```python
from build123d import *

# Parameters (mm, degrees)
SKETCH1_R               = 33
SKETCH1_R_2             = 25.5
BOSS_EXTRUDE2_DEPTH     = 17
BOSS_EXTRUDE3_START     = -5
SKETCH1_3_R             = 33
BOSS_EXTRUDE3_DEPTH     = 5
CUT_EXTRUDE4_DEPTH      = 50.668903753
CUT_EXTRUDE4_DEPTH_BACK = 3
SKETCH1_5_R             = 1.5
CUT_EXTRUDE6_DEPTH      = 50.668903753
CUT_EXTRUDE6_DEPTH_BACK = 50.668903753
SKETCH3_R               = 1.7
SKETCH3_R_2             = 3.5
SKETCH4_R               = 10
CUT_EXTRUDE7_DEPTH      = 2
SKETCH6_R               = 1.7
CUT_EXTRUDE8_DEPTH      = 10
SKETCH7_R               = 2.75
CUT_EXTRUDE9_DEPTH      = 2


with BuildPart() as part:
    # Sketch1 → Boss-Extrude2 (new body)
    with BuildSketch(Plane.XY):
        Circle(SKETCH1_R)
        Circle(SKETCH1_R_2, mode=Mode.SUBTRACT)
    extrude(amount=BOSS_EXTRUDE2_DEPTH)

    # Sketch1<3> → Boss-Extrude3 (add)
    with BuildSketch(Plane.XY.offset(BOSS_EXTRUDE3_START)):
        Circle(SKETCH1_3_R)
    extrude(amount=BOSS_EXTRUDE3_DEPTH)

    # Sketch1<5> → Cut-Extrude4 (cut, two sides: drawn at the far end of the back side and taken through both)
    with BuildSketch(Plane.XY.offset(-CUT_EXTRUDE4_DEPTH_BACK)):
        with Locations(Location((25, 0, 0), (0, 0, 72.141537302))):
            Circle(SKETCH1_5_R)
        with Locations(Location((24.273545436, -5.982891607, 0), (0, 0, 274.012308852))):
            Circle(SKETCH1_5_R)
        with Locations(Location((22.136400641, -11.618079301, 0), (0, 0, 260.166155006))):
            Circle(SKETCH1_5_R)
        with Locations(Location((18.712768704, -16.578066456, 0), (0, 0, 246.32000116))):
            Circle(SKETCH1_5_R)
        with Locations(Location((14.201618668, -20.574596647, 0), (0, 0, 232.473847314))):
            Circle(SKETCH1_5_R)
        with Locations(Location((8.865122176, -23.375406067, 0), (0, 0, 218.627693468))):
            Circle(SKETCH1_5_R)
        with Locations(Location((3.013417006, -24.817721852, 0), (0, 0, 204.781539621))):
            Circle(SKETCH1_5_R)
        with Locations(Location((-3.013417006, -24.817721852, 0), (0, 0, 190.935385775))):
            Circle(SKETCH1_5_R)
        with Locations(Location((-8.865122176, -23.375406067, 0), (0, 0, 177.089231929))):
            Circle(SKETCH1_5_R)
        with Locations(Location((-14.201618668, -20.574596647, 0), (0, 0, 163.243078083))):
            Circle(SKETCH1_5_R)
        with Locations(Location((-18.712768704, -16.578066456, 0), (0, 0, 149.396924237))):
            Circle(SKETCH1_5_R)
        with Locations(Location((-22.136400641, -11.618079301, 0), (0, 0, 135.550770391))):
            Circle(SKETCH1_5_R)
        with Locations(Location((-24.273545436, -5.982891607, 0), (0, 0, 121.704616545))):
            Circle(SKETCH1_5_R)
        with Locations(Location((-25, 0, 0), (0, 0, 107.858462698))):
            Circle(SKETCH1_5_R)
        with Locations(Location((-24.273545436, 5.982891607, 0), (0, 0, 238.295383455))):
            Circle(SKETCH1_5_R)
        with Locations(Location((-22.136400641, 11.618079301, 0), (0, 0, 224.449229609))):
            Circle(SKETCH1_5_R)
        with Locations(Location((-18.712768704, 16.578066456, 0), (0, 0, 210.603075763))):
            Circle(SKETCH1_5_R)
        with Locations(Location((-14.201618668, 20.574596647, 0), (0, 0, 196.756921917))):
            Circle(SKETCH1_5_R)
        with Locations(Location((-8.865122176, 23.375406067, 0), (0, 0, 182.910768071))):
            Circle(SKETCH1_5_R)
        with Locations(Location((-3.013417006, 24.817721852, 0), (0, 0, 169.064614225))):
            Circle(SKETCH1_5_R)
        with Locations(Location((3.013417006, 24.817721852, 0), (0, 0, 155.218460378))):
            Circle(SKETCH1_5_R)
        with Locations(Location((8.865122176, 23.375406067, 0), (0, 0, 141.372306532))):
            Circle(SKETCH1_5_R)
        with Locations(Location((14.201618668, 20.574596647, 0), (0, 0, 127.526152686))):
            Circle(SKETCH1_5_R)
        with Locations(Location((18.712768704, 16.578066456, 0), (0, 0, 113.67999884))):
            Circle(SKETCH1_5_R)
        with Locations(Location((22.136400641, 11.618079301, 0), (0, 0, 99.833844994))):
            Circle(SKETCH1_5_R)
        with Locations(Location((24.273545436, 5.982891607, 0), (0, 0, 85.987691148))):
            Circle(SKETCH1_5_R)
    extrude(amount=CUT_EXTRUDE4_DEPTH + CUT_EXTRUDE4_DEPTH_BACK, mode=Mode.SUBTRACT)

    # Sketch3 → Cut-Extrude6 (cut, two sides: drawn at the far end of the back side and taken through both)
    with BuildSketch(Plane.XY.offset(-CUT_EXTRUDE6_DEPTH_BACK)):
        with Locations((0, 29.5)):
            Circle(SKETCH3_R)
        with Locations((29.5, 0)):
            Circle(SKETCH3_R)
        with Locations((0, -29.5)):
            Circle(SKETCH3_R)
        with Locations((-29.5, 0)):
            Circle(SKETCH3_R)
        Circle(SKETCH3_R_2)
    extrude(amount=CUT_EXTRUDE6_DEPTH + CUT_EXTRUDE6_DEPTH_BACK, mode=Mode.SUBTRACT)

    # Sketch4 → Cut-Extrude7 (cut)
    with BuildSketch(Plane(origin=(0, 0, -5), x_dir=(-1, 0, 0), z_dir=(0, 0, -1))):
        Circle(SKETCH4_R)
    extrude(amount=-CUT_EXTRUDE7_DEPTH, mode=Mode.SUBTRACT)

    # Sketch6 → Cut-Extrude8 (cut)
    with BuildSketch(Plane.XY.offset(17)):
        with Locations((-20.859650045, 20.859650045)):
            Circle(SKETCH6_R)
        with Locations((20.859650045, 20.859650045)):
            Circle(SKETCH6_R)
        with Locations((20.859650045, -20.859650045)):
            Circle(SKETCH6_R)
        with Locations((-20.859650045, -20.859650045)):
            Circle(SKETCH6_R)
    extrude(amount=-CUT_EXTRUDE8_DEPTH, mode=Mode.SUBTRACT)

    # Sketch7 → Cut-Extrude9 (cut)
    with BuildSketch(Plane.XY.offset(17)):
        with Locations((0, 29.5)):
            Circle(SKETCH7_R)
        with Locations((29.5, 0)):
            Circle(SKETCH7_R)
        with Locations((0, -29.5)):
            Circle(SKETCH7_R)
        with Locations((-29.5, 0)):
            Circle(SKETCH7_R)
    extrude(amount=-CUT_EXTRUDE9_DEPTH, mode=Mode.SUBTRACT)


solid = part.part
```
Can you work these out from the model? Positions are in its coordinate system, mm. A direction names the side the tool comes from. Coordinates: 2 decimals unless noted, no trailing zeros. Write each loop counter-clockwise with the first axis right and the second up, starting at its lowest first coordinate (ties: lowest second). Pieces come first, ordered by that corner, then holes. Notation, with made-up numbers: (47.25, 57.5) - (56.25, 57.5) arc R27 ccw to (56.25, 93.5) - close; hole circle Ø7 at (0.25, 34.5). An arc over 180 degrees is marked (long way). Return JSON: item names as keys, results as strings.
Q1. If we section it at B-B (x = 29.5): Please give me the cut outline in (y, z), then the cut area to 3 significant figures.
Computed values:
{"outline": "(-14.79, -5) - (-1.7, -5) - (-1.7, 15) - (-2.75, 15) - (-2.75, 17) - (-14.79, 17) - close; (1.7, -5) - (14.79, -5) - (14.79, 17) - (2.75, 17) - (2.75, 15) - (1.7, 15) - close", "area": "572 mm2"}
Q2. On a 3-axis mill with a long thin cutter (end or side, diameter ignored), from which of +Z, -Z, +X, -X, +Y, -Y can I reach the whole of each face in a straight line? I mean faces 1 (the flat face through (22, 12, -3)), 2 (the cylindrical face through (-0.37, 27.84, 4.86)). Say none if no direction works.
Computed values:
{"face 1": "+Z", "face 2": "+Z, -Z"}
Q3. I'm going to push flat-ended pins straight in: pin 1 Ø0.9 at (x, y) = (18, 16.5) entering from +Z; pin 2 Ø5 at (y, z) = (-23.5, 0.5) entering from -X; pin 3 Ø12 at (x, z) = (-20, 11) entering from -Y. Where does each tip first touch, or does it pass through?
Computed values:
{"pin 1": "stops at z = -3", "pin 2": "stops at x = -25.46", "pin 3": "stops at y = -29.88"}
Q4. Please list where these lines run through material, in increasing order: L1, parallel to Y at x = 0, z = 6.25; L2, parallel to X at y = -21, z = 11; L3, parallel to X at y = 1, z = 15.5. Write a range as from..to.
Computed values:
{"L1": "y = -33..-31.2, -27.8..-25.5, 25.5..27.8, 31.2..33", "L2": "x = -25.46..-22.55, -19.17..-15.64, 15.64..19.17, 22.55..25.46", "L3": "x = -32.98..-32.06, -26.94..-26.12, 26.12..26.94, 32.06..32.98"}
Q5. If we section it at A-A (x = -0.5): Count the separate pieces of the cut face and the enclosed holes in it, then the cut area to 3 significant figures.
Computed values:
{"separate pieces": "4", "enclosed holes": "0", "area": "373 mm2"}
